Verification items for the finished model (mm, model axes). A direction names the side the tool comes from. Give positions to 0.01 mm unless a question says otherwise; leave off trailing zeros. Write each loop counter-clockwise with the first axis right and the second up, starting at its lowest first coordinate (ties: lowest second). Pieces come first, ordered by that corner, then holes. Notation, with made-up numbers: (20.5, -30.75) - (39.5, -30.75) arc R22 cw to (39.5, -1.75) - close; hole circle Ø3 at (50.25, -27). An arc over 180 degrees is marked (long way). Answer as a JSON object with one key per item and string values. Group by question number.
Item 1: Tool access check on faces 1 (the face through (0, -104, 0)), 2 (the face through (-2.17, -49.37, -9.76)). Record the directions out of +Z, -Z, +X, -X, +Y, -Y that give a thin tool (end or side, any length) a straight path to the whole face; none if there is none.
Item 2: Sectioned sample at A-A, the plane y = -48. Record the boundary of the cut face in (x, z).
Item 3: Scan lines: line 1 along Y through (x, z) = (-12, 3); line 2 along X through (y, z) = (-40, -4.5); line 3 along X through (y, z) = (-25.5, 0.5). Record each from-to range of solid material in increasing order. Write a range as [from, to].
Item 4: Go/stop test with flat-tipped pins: pin 1 (1.5 mm diameter, centred on x = -4.5, y = -46, fed in from -Z); pin 2 (12 mm diameter, centred on x = -11, z = -8.5, fed in from +Y); pin 3 (1.5 mm diameter, centred on x = 1.5, y = -47, fed in from -Z). Record where each tip stops, or that it passes through.
```python
from build123d import *

# Parameters (mm, degrees)
F0_R     = 10
F1_DEPTH = 104
F2_R     = 15
F3_DEPTH = 4
F4_R     = 4.99999


# Not quite as in the source:
# - a fillet or chamfer that OpenCascade refuses, or shapes differently, is made with other operations: its cross-section is extruded or revolved along the edge and cut away or added
# - a fillet or chamfer is up to 0.001 mm smaller than in the source, because OpenCascade refuses the exact size


with BuildPart() as f1:
    # F0 (on Front) → F1 (new body)
    with BuildSketch(Plane.XZ):
        Circle(F0_R)
    extrude(amount=F1_DEPTH)

    # F2 (on face) → F3 (join)
    with BuildSketch(Plane.XZ.offset(104)):
        Circle(F2_R)
    extrude(amount=-F3_DEPTH)

    # F4 (radius 5 in the source; OpenCascade refuses exactly that, so slightly less here)
    f4_edges = [f1.edges().sort_by_distance(p)[0] for p in [
        (-10, -100, 0),
    ]]
    fillet(f4_edges, radius=F4_R)

    # F5: fillet of radius 5 on 2 edges, made by hand

    # F5_s1 → F5_t2 (revolve, cut)
    with BuildSketch(Plane.XY):
        with BuildLine():
            ThreePointArc((15, -100), (13.2632981746, -102.8729833462), (10.1010205144, -104))
            Line((10.1010205144, -104), (15, -104))
            Line((15, -104), (15, -100))
        make_face()
    revolve(axis=Axis((0, -104, 0), (0, -1, 0)), mode=Mode.SUBTRACT)

    # F5_s3 → F5_t4 (revolve, cut)
    with BuildSketch(Plane.XY):
        with BuildLine():
            ThreePointArc((10, -5), (8.5355339059, -1.4644660941), (5, 0))
            Line((5, 0), (10, 0))
            Line((10, 0), (10, -5))
        make_face()
    revolve(axis=Axis((0, 0, 0), (0, -1, 0)), mode=Mode.SUBTRACT)


solid = f1.part
```
Geometry check:
{
 "1": {"face 1": "+Z, -Z, +X, -X, -Y", "face 2": "+Y"},
 "2": {"outline": "circle Ø20 at (0, 0)"},
 "3": {"line 1": "[-103.46, -99.25]", "line 2": "[-8.93, 8.93]", "line 3": "[-9.99, 9.99]"},
 "4": {"pin 1": "z = -9.27", "pin 2": "y = -0.93", "pin 3": "z = -9.97"}
}
